Can you work these out from the drawing? Everything is in mm from the part's minimum corner. A direction names the side the tool comes from. Coordinates: 2 decimals unless noted, no trailing zeros. Loops run counter-clockwise (first coordinate to the right, second up) from the corner with the lowest first, then second, coordinate; pieces in that order, holes last.
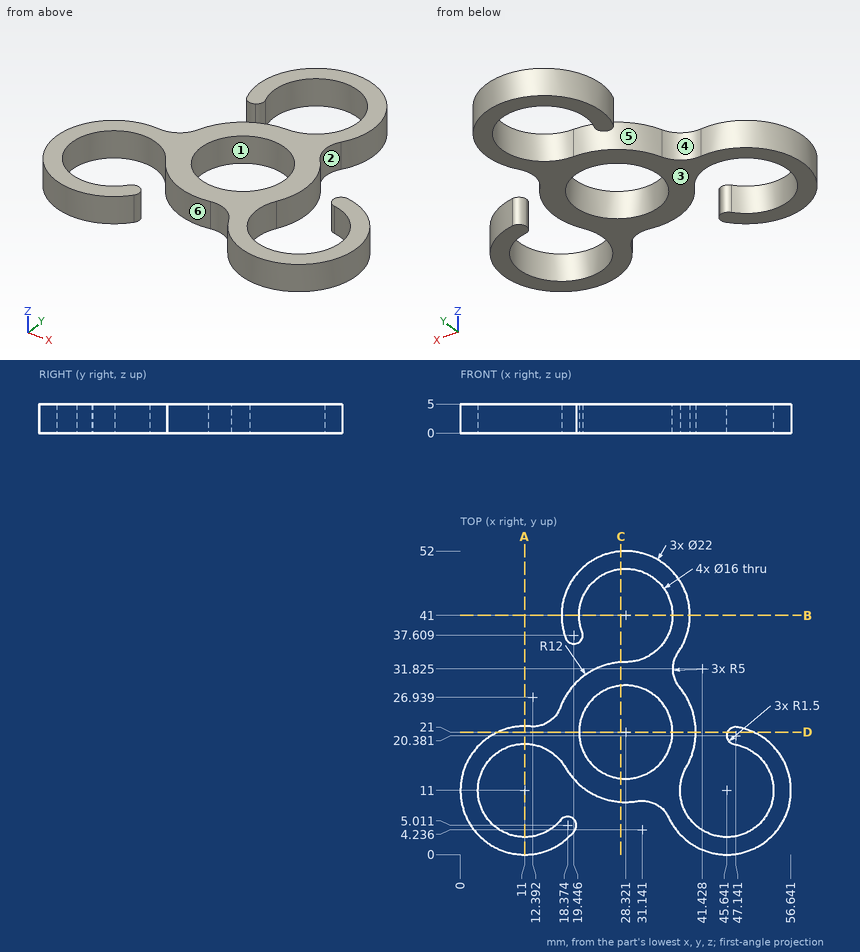
Item 1: I'm going to push flat-ended pins straight in: P1, Ø1.5, axis at y = 5.5, z = 3, coming from the +X side; P2, Ø6, axis at x = 25.5, y = 25, coming from the -Z side; P3, Ø1, axis at y = 45.5, z = 0.5, coming from the +X side; P4, Ø1, axis at x = 30.5, z = 3, coming from the -Y side. Where does each tip first touch, or does it pass through?
Results are:
P1: stops at x = 55.56
P2: passes through
P3: stops at x = 38.57
P4: stops at y = 9.12
Item 2: I need wall thicknesses on line 1 along X through (y, z) = (41, 1.8); line 2 along Y through (x, z) = (10.5, 0.3) (1 decimal); line 3 along X through (y, z) = (11, 2.8) (1 decimal). Which ranges of each line are inside material? Lowest first, please.
Results are:
line 1: x = 17.32 to 20.32, 36.32 to 39.32
line 2: y = 0 to 3, 19 to 22
line 3: x = 0 to 3, 21.7 to 37.6, 53.6 to 56.6
Item 3: On a 3-axis mill with a long thin cutter (end or side, diameter ignored), from which of +Z, -Z, +X, -X, +Y, -Y can I reach the whole of each face in a straight line? I mean the marked faces 4, 5 and 6. Say none if no direction works.
Results are:
face 4: +Z, -Z, +Y
face 5: +Z, -Z, -X
face 6: +Z, -Z
Item 4: Suppose I cut it at C-C, the plane x = 27.5. Please give me the cut outline in (y, z).
Results are:
outline: (9.03, 0) - (13.04, 0) - (13.04, 5) - (9.03, 5) - close; (28.96, 0) - (32.97, 0) - (32.97, 5) - (28.96, 5) - close; (48.96, 0) - (51.97, 0) - (51.97, 5) - (48.96, 5) - close
Item 5: We'd pull the mould along X, two halves only. Please class the marked faces 1, 2 and 3: +X half, -X half, draft (parallel to the pull), parting line (faces both ways), or undercut.
Results are:
face 1: undercut
face 2: +X half
face 3: draft
Item 6: Suppose I cut it at A-A, the plane x = 11. Please give me the cut outline in (y, z).
Results are:
outline: (0, 0) - (3, 0) - (3, 5) - (0, 5) - close; (19, 0) - (22, 0) - (22, 5) - (19, 5) - close
Item 7: Suppose I cut it at B-B, the plane y = 41. Please give me the cut outline in (x, z).
Results are:
outline: (17.32, 0) - (20.32, 0) - (20.32, 5) - (17.32, 5) - close; (36.32, 0) - (39.32, 0) - (39.32, 5) - (36.32, 5) - close
Item 8: Suppose I cut it at D-D, the plane y = 21. Please give me the cut outline in (x, z) (1 decimal), plus the area to 3 significant figures.
Results are:
outline: (6.4, 0) - (20.3, 0) - (20.3, 5) - (6.4, 5) - close; (36.3, 0) - (40.3, 0) - (40.3, 5) - (36.3, 5) - close; (45.8, 0) - (50.2, 0) - (50.2, 5) - (45.8, 5) - close
area: 112 mm2
